Input: part model. Units: mm. Frame: model coordinates. A direction names the side the tool comes from. Round coordinates to 2 decimals unless told otherwise and drop trailing zeros. Write each loop counter-clockwise with the first axis right and the second up, starting at its lowest first coordinate (ties: lowest second). Pieces come first, ordered by that corner, then holes. Notation, with made-up numbers: (47, 64) -> (69, 64) arc R33 cw to (69, 93) -> close; hole circle Ø8 at (8.25, 35). An arc over 180 degrees is marked (long way). Write item = value, one per line.
```python
from build123d import *

# Parameters (mm, degrees)
SKETCH1_3_W         = 80
SKETCH1_3_H         = 80
SKETCH1_3_R         = 15
SKETCH1_3_R_2       = 2.5
BOSS_EXTRUDE3_DEPTH = 5
BOSS_EXTRUDE4_START = 5
SKETCH1_W           = 80
SKETCH1_H           = 80
SKETCH1_R           = 2.5
SKETCH1_R_2         = 25
BOSS_EXTRUDE4_DEPTH = 5
CUT_EXTRUDE1_DEPTH  = 90.582364336
CUT_EXTRUDE2_DEPTH  = 90.582364475
CUT_EXTRUDE3_START  = -80
CUT_EXTRUDE3_DEPTH  = 80


# Read off the part's stored shape, not the designer's step: Cut-Extrude3
with BuildPart() as part:
    # Sketch1_3 → Boss-Extrude3 (new body)
    with BuildSketch(Plane(origin=(0, 0, 0), x_dir=(1, 0, 0), z_dir=(0, 1, 0))):
        Rectangle(SKETCH1_3_W, SKETCH1_3_H)
        with Locations(Location((0, 0, 0), (0, 0, 270))):
            Circle(SKETCH1_3_R, mode=Mode.SUBTRACT)
        with Locations(Location((-32, 32, 0), (0, 0, 270))):
            Circle(SKETCH1_3_R_2, mode=Mode.SUBTRACT)
        with Locations(Location((-32, -32, 0), (0, 0, 270))):
            Circle(SKETCH1_3_R_2, mode=Mode.SUBTRACT)
        with Locations(Location((32, -32, 0), (0, 0, 270))):
            Circle(SKETCH1_3_R_2, mode=Mode.SUBTRACT)
        with Locations(Location((32, 32, 0), (0, 0, 270))):
            Circle(SKETCH1_3_R_2, mode=Mode.SUBTRACT)
    extrude(amount=-BOSS_EXTRUDE3_DEPTH)

    # Sketch1 → Boss-Extrude4 (add)
    with BuildSketch(Plane(origin=(0, 0, 0), x_dir=(1, 0, 0), z_dir=(0, 1, 0)).offset(BOSS_EXTRUDE4_START)):
        Rectangle(SKETCH1_W, SKETCH1_H)
        with Locations(Location((-32, -32, 0), (0, 0, 270))):
            Circle(SKETCH1_R, mode=Mode.SUBTRACT)
        with Locations(Location((32, -32, 0), (0, 0, 270))):
            Circle(SKETCH1_R, mode=Mode.SUBTRACT)
        with Locations(Location((0, 0, 0), (0, 0, 270))):
            Circle(SKETCH1_R_2, mode=Mode.SUBTRACT)
        with Locations(Location((-32, 32, 0), (0, 0, 270))):
            Circle(SKETCH1_R, mode=Mode.SUBTRACT)
        with Locations(Location((32, 32, 0), (0, 0, 270))):
            Circle(SKETCH1_R, mode=Mode.SUBTRACT)
    extrude(amount=-BOSS_EXTRUDE4_DEPTH)

    # Sketch5 → Cut-Extrude1 (cut, through all)
    with BuildSketch(Plane(origin=(0, 0, -40), x_dir=(-1, 0, 0), z_dir=(0, 0, -1))):
        with BuildLine():
            Line((40, 5), (-40, 5))
            ThreePointArc((-40, 5), (0, 1.779253585), (40, 5))
        make_face()
    extrude(amount=-CUT_EXTRUDE1_DEPTH, mode=Mode.SUBTRACT)

    # Sketch7 → Cut-Extrude2 (cut, through all)
    with BuildSketch(Plane(origin=(40, 0, 0), x_dir=(0, 0, -1), z_dir=(1, 0, 0))):
        with BuildLine():
            ThreePointArc((0, -5), (-20.059793007, -4.225007869), (-40, -1.904651573))
            Line((-40, -1.904651573), (-40, -5))
            Line((-40, -5), (0, -5))
        make_face()
    extrude(amount=-CUT_EXTRUDE2_DEPTH, mode=Mode.SUBTRACT)

    # Cut-Extrude3 outline → Cut-Extrude3 (cut)
    with BuildSketch(Plane(origin=(40, 0, 0), x_dir=(0, 0, -1), z_dir=(1, 0, 0)).offset(CUT_EXTRUDE3_START)):
        with BuildLine():
            ThreePointArc((40, -1.904651573), (20.059793007, -4.225007869), (0, -5))
            Line((0, -5), (40, -5))
            Line((40, -5), (40, -1.904651573))
        make_face()
    extrude(amount=CUT_EXTRUDE3_DEPTH, mode=Mode.SUBTRACT)


solid = part.part
```
1) Cut plane D-D (z = 32). Return the cut outline in (x, y).
Solutions:
outline = (-40, -3.02) -> (-34.5, -3.02) -> (-34.5, 4.17) arc R250 cw to (-40, 5) -> close; (-29.5, -3.02) -> (29.5, -3.02) -> (29.5, 3.53) arc R250 cw to (-29.5, 3.53) -> close; (34.5, -3.02) -> (40, -3.02) -> (40, 5) arc R250 cw to (34.5, 4.17) -> close
2) Line query: L1, parallel to Z at x = -32, y = 1.75; L2, parallel to Z at x = -33.5, y = 2.25. Output: solid intervals per line, ascending. Write a range as from..to.
Solutions:
L1 = -40..-34.5, -29.5..29.5, 34.5..40
L2 = -40..-34, -30..30, 34..40
3) Cut plane A-A (z = -2). Return the cut outline in (x, y).
Solutions:
outline = (-40, -4.99) -> (-14.87, -4.99) -> (-14.87, 0) -> (-24.92, 0) -> (-24.92, 3.02) arc R250 cw to (-40, 5) -> close; (14.87, -4.99) -> (40, -4.99) -> (40, 5) arc R250 cw to (24.92, 3.02) -> (24.92, 0) -> (14.87, 0) -> close
4) Access query for faces 5 (the face through (11, 0, 11)), 6 (the face through (18.4, 2.457, -18.338)). Directions: +Z, -Z, +X, -X, +Y, -Y. A direction counts if a zero-diameter tool reaches every point of the face in a straight line with its end or side. Return the directions, or none.
Solutions:
face_5 = +Y
face_6 = +Z, -Z, +Y
5) Cut plane C-C (x = -33). Return the cut outline in (y, z), and give its area (3 significant figures).
Solutions:
outline = (-3.3, -29.71) -> (3.97, -29.71) -> (3.97, 29.71) -> (-3.3, 29.71) arc R260 ccw to start; (-2.73, -34.29) arc R260 ccw to (-1.9, -40) -> (3.97, -40) -> (3.97, -34.29) -> close; (-2.73, 34.29) -> (3.97, 34.29) -> (3.97, 40) -> (-1.9, 40) arc R260 ccw to start
area = 571 mm^2
6) Cut plane B-B (x = -6.5). Return the cut outline in (y, z).
Solutions:
outline = (-4.65, -13.52) arc R260 ccw to (-1.9, -40) -> (1.86, -40) -> (1.86, -24.14) -> (0, -24.14) -> (0, -13.52) -> close; (-4.65, 13.52) -> (0, 13.52) -> (0, 24.14) -> (1.86, 24.14) -> (1.86, 40) -> (-1.9, 40) arc R260 ccw to start
7) First-contact query: P1, Ø1.5, axis at x = 2, z = -30.5, coming from the -Y side; P2, Ø3, axis at x = 32, z = -32, coming from the -Y side; P3, Ø5, axis at x = -10, z = 29, coming from the +Y side; P4, Ø5, axis at x = 15, y = 3, coming from the +Z side. Flat tips, straight axial feed; report the tip coordinate or a pass-through.
Solutions:
P1 = -3.29
P2 = through
P3 = 2.09
P4 = 40
8) Draft query along X for faces 1 (the face through (40, 0, 1)), 2 (the face through (0.66, -2.465, -14.985)), 3 (the face through (-40, 0, 1)), 4 (the face through (-33.5, 0.5, 30)). Return one class per face: +X half, -X half, draft (parallel to the pull), parting line (faces both ways), or undercut.
Solutions:
face_1 = +X half
face_2 = undercut
face_3 = -X half
face_4 = undercut
